from build123d import *

# Parameters (mm, degrees)
SKETCH1_W           = 25.4
SKETCH1_H           = 50.8
SKETCH1_W_2         = 20.32
SKETCH1_H_2         = 45.72
BOSS_EXTRUDE1_DEPTH = 584.2
SKETCH2_R           = 2.032
CUT_EXTRUDE1_DEPTH  = 587.542044529
SKETCH3_R           = 2.032
CUT_EXTRUDE2_DEPTH  = 586.303305988


with BuildPart() as part:
    # Sketch1 → Boss-Extrude1 (new body)
    with BuildSketch(Plane(origin=(0, 0, 0), x_dir=(1, 0, 0), z_dir=(0, 1, 0))):
        Rectangle(SKETCH1_W, SKETCH1_H)
        Rectangle(SKETCH1_W_2, SKETCH1_H_2, mode=Mode.SUBTRACT)
    extrude(amount=BOSS_EXTRUDE1_DEPTH)

    # Sketch2 → Cut-Extrude1 (cut, through all)
    with BuildSketch(Plane.XY.offset(25.4)):
        Circle(SKETCH2_R)
        with Locations((0, 25.4)):
            Circle(SKETCH2_R)
        with Locations((0, 50.8)):
            Circle(SKETCH2_R)
        with Locations((0, 76.2)):
            Circle(SKETCH2_R)
        with Locations((0, 101.6)):
            Circle(SKETCH2_R)
        with Locations((0, 127)):
            Circle(SKETCH2_R)
        with Locations((0, 152.4)):
            Circle(SKETCH2_R)
        with Locations((0, 177.8)):
            Circle(SKETCH2_R)
        with Locations((0, 203.2)):
            Circle(SKETCH2_R)
        with Locations((0, 228.6)):
            Circle(SKETCH2_R)
        with Locations((0, 254)):
            Circle(SKETCH2_R)
        with Locations((0, 279.4)):
            Circle(SKETCH2_R)
        with Locations((0, 304.8)):
            Circle(SKETCH2_R)
        with Locations((0, 330.2)):
            Circle(SKETCH2_R)
        with Locations((0, 355.6)):
            Circle(SKETCH2_R)
        with Locations((0, 381)):
            Circle(SKETCH2_R)
        with Locations((0, 406.4)):
            Circle(SKETCH2_R)
        with Locations((0, 431.8)):
            Circle(SKETCH2_R)
        with Locations((0, 457.2)):
            Circle(SKETCH2_R)
        with Locations((0, 482.6)):
            Circle(SKETCH2_R)
        with Locations((0, 508)):
            Circle(SKETCH2_R)
        with Locations((0, 533.4)):
            Circle(SKETCH2_R)
        with Locations((0, 558.8)):
            Circle(SKETCH2_R)
        with Locations((0, 584.2)):
            Circle(SKETCH2_R)
    extrude(amount=-CUT_EXTRUDE1_DEPTH, mode=Mode.SUBTRACT)

    # Sketch3 → Cut-Extrude2 (cut, through all)
    with BuildSketch(Plane.ZY.offset(12.7)):
        with Locations((0, 520.7)):
            Circle(SKETCH3_R)
        with Locations((0, 508)):
            Circle(SKETCH3_R)
        with Locations((0, 495.3)):
            Circle(SKETCH3_R)
        with Locations((0, 482.6)):
            Circle(SKETCH3_R)
        with Locations((0, 469.9)):
            Circle(SKETCH3_R)
    extrude(amount=-CUT_EXTRUDE2_DEPTH, mode=Mode.SUBTRACT)


solid = part.part
CAD build for the part. Positions are in the model's coordinates, mm. A direction names the side the tool comes from. Coordinates: 2 decimals unless noted, no trailing zeros. Write each loop counter-clockwise with the first axis right and the second up, starting at its lowest first coordinate (ties: lowest second). Pieces come first, ordered by that corner, then holes. Notation, with made-up numbers: M 70.5,-37 L 122.5,-37 A34 ccw 122.5,-4 Z; hole C 48,50.5 d9. An arc over 180 degrees is marked long. Answer as a JSON object with one key per item and string values. Group by question number.
1) Saw through at A-A (z = -8). Write the cut outline in (x, y), plus the area to 3 significant figures.
2) Wall check: line 1 (X direction, y = 42, z = 7.5); line 2 (Z direction, x = 7, y = 197); line 3 (Z direction, x = -11.65, y = 508). Give the ranges that are in metal, low to high. Write a range as from..to.
3) Mould opens along Z. For faces 3 (the face through (-12.7, 288, 0)), 4 (the face through (0, 288, 22.86)), 5 (the face through (0, 288, -25.4)) say: +Z half, -Z half, draft (parallel to the pull), parting line (faces both ways), or undercut.
4) Pin check, flat tip, straight feed: pin 1 Ø2.5 at (x, y) = (0, 355.6) entering from -Z. Stop position of the tip, or through.
5) Tool access for faces 1 (the face through (-10.16, 288, 0)), 2 (the face through (11, 584.2, 0)): list every direction of +Z, -Z, +X, -X, +Y, -Y with a clear straight run to the whole face (end or side of a thin tool).
6) Saw through at B-B (y = 319). Write the cut outline in (x, z).
Values follow:
{
 "1": {"outline": "M -12.7,0 L -10.16,0 L -10.16,584.2 L -12.7,584.2 Z; M 10.16,0 L 12.7,0 L 12.7,584.2 L 10.16,584.2 Z", "area": "2,970 mm2"},
 "2": {"line 1": "x = -12.7..-10.16, 10.16..12.7", "line 2": "z = -25.4..-22.86, 22.86..25.4", "line 3": "z = -25.4..-2.03, 2.03..25.4"},
 "3": {"face 3": "draft", "face 4": "undercut", "face 5": "-Z half"},
 "4": {"pin 1": "passes through"},
 "5": {"face 1": "+Y, -Y", "face 2": "+Z, -Z, +X, -X, +Y"},
 "6": {"outline": "M -12.7,-25.4 L 12.7,-25.4 L 12.7,25.4 L -12.7,25.4 Z; hole M -10.16,-22.86 L 10.16,-22.86 L 10.16,22.86 L -10.16,22.86 Z"}
}
